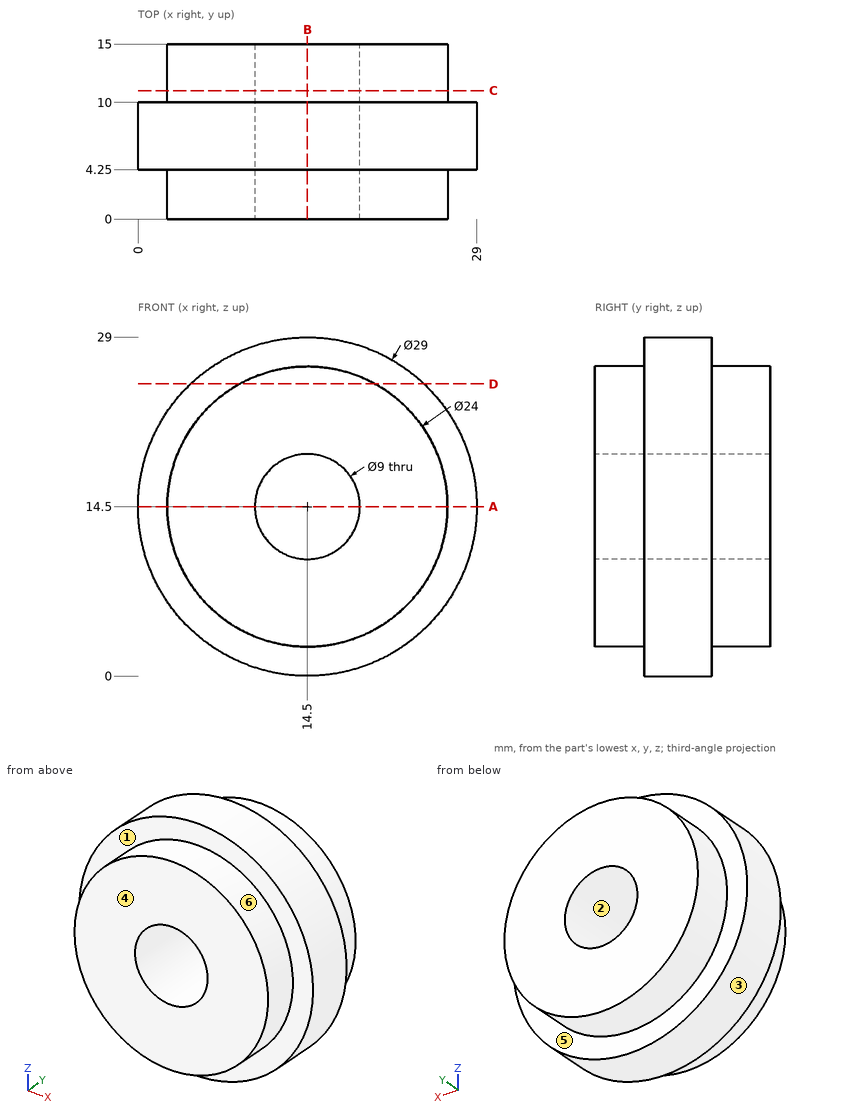
The drawing under review shows one solid part. Ordinate dimensions are in mm from its lowest x, y, z. A direction names the side the tool comes from. Give positions to 0.01 mm unless a question says otherwise; leave off trailing zeros. Write each loop counter-clockwise with the first axis right and the second up, starting at its lowest first coordinate (ties: lowest second). Pieces come first, ordered by that corner, then holes.
1. Add section C-C, the plane y = 11. Write out the cut boundary in (x, z), plus the area to 3 significant figures.
2. Add section A-A, the plane z = 14.5. Write out the cut boundary in (x, y).
3. Add section D-D, the plane z = 25. Write out the cut boundary in (x, y), plus the area to 3 significant figures.
4. Wall thickness on L1, parallel to Z at x = 14.5, y = 12.25; L2, parallel to Z at x = 14.5, y = 4.5; L3, parallel to Y at x = 6, z = 23: over which ranges is each line inside the solid? List them lowest first.
5. For P1, Ø14.5, axis at x = 11, z = 19, coming from the -Y side; P2, Ø1.5, axis at y = 3, z = 22, coming from the -X side; P3, Ø2, axis at y = 9, z = 11.5, coming from the -X side; P4, Ø1.5, axis at x = 16.5, y = 9.5, coming from the +Z side, all flat-tipped, find the tip position at first contact; note any pin that passes through.
6. Add section B-B, the plane x = 14.5. Write out the cut boundary in (y, z).
7. Tool access review of the marked faces 4, 5 and 6: name each direction out of +Z, -Z, +X, -X, +Y, -Y from which nothing blocks a thin tool from reaching the whole face with its end or side.
8. Draft analysis for pull direction X (two halves, no side actions). For the marked faces 1, 2 and 3, state which applies: +X half, -X half, draft (parallel to the pull), parting line (faces both ways), or undercut.
Worked answers:
1. outline: circle Ø24 at (14.5, 14.5); hole circle Ø9 at (14.5, 14.5)
1. area: 389 mm2
2. outline: (0, 4.25) - (2.5, 4.25) - (2.5, 0) - (10, 0) - (10, 15) - (2.5, 15) - (2.5, 10) - (0, 10) - close; (19, 0) - (26.5, 0) - (26.5, 4.25) - (29, 4.25) - (29, 10) - (26.5, 10) - (26.5, 15) - (19, 15) - close
3. outline: (4.5, 4.25) - (8.69, 4.25) - (8.69, 0) - (20.31, 0) - (20.31, 4.25) - (24.5, 4.25) - (24.5, 10) - (20.31, 10) - (20.31, 15) - (8.69, 15) - (8.69, 10) - (4.5, 10) - close
3. area: 222 mm2
4. L1: z = 2.5 to 10, 19 to 26.5
4. L2: z = 0 to 10, 19 to 29
4. L3: y = 4.25 to 10
5. P1: stops at y = 0
5. P2: stops at x = 4.58
5. P3: stops at x = 0.14
5. P4: stops at z = 28.95
6. outline: (0, 2.5) - (4.25, 2.5) - (4.25, 0) - (10, 0) - (10, 2.5) - (15, 2.5) - (15, 10) - (0, 10) - close; (0, 19) - (15, 19) - (15, 26.5) - (10, 26.5) - (10, 29) - (4.25, 29) - (4.25, 26.5) - (0, 26.5) - close
7. face 4: +Z, -Z, +X, -X, -Y
7. face 5: +Y
7. face 6: -Y
8. face 1: draft
8. face 2: undercut
8. face 3: parting line
